Geometry: final body of the model. Coordinates: model frame, mm. A direction names the side the tool comes from. Give positions to 0.01 mm unless a question says otherwise; leave off trailing zeros. Loops run counter-clockwise (first coordinate to the right, second up) from the corner with the lowest first, then second, coordinate; pieces in that order, holes last. Notation, with made-up numbers: (54, 8) -> (111, 8) arc R25 cw to (111, 40) -> close; hole circle Ø4 at (-19.5, 64). An arc over 180 degrees is marked (long way). Answer in a Markdown table with one row per item. Add a question column.
1) Section query B-B (y = -2). Return the cut outline in (x, z), plus the area to 3 significant figures.
2) Section query D-D (y = 3.75). Return the cut outline in (x, z).
3) Section query A-A (z = 0). Return the cut outline in (x, y).
4) Draft query along X for faces 5 (the cylindrical face through (-0.217, 4.205, -7.276)), 6 (the flat face through (-1, 0, -8.9)), 7 (the cylindrical face through (-1.5, 0.04, 0.07)). Return one class per face: +X half, -X half, draft (parallel to the pull), parting line (faces both ways), or undercut.
5) Access query for faces 1 (the cylindrical face through (-0.217, -4.245, -7.276)), 2 (the flat face through (3, 0, -1)), 3 (the flat face through (1, 0, -10)), 4 (the flat face through (0, 0, 8)). Directions: +Z, -Z, +X, -X, +Y, -Y. A direction counts if a zero-diameter tool reaches every point of the face in a straight line with its end or side. Return the directions, or none.
6) Line query: line 1 (Y direction, x = -0.35, z = -1.5); line 2 (Z direction, x = -0.7, y = -0.75); line 3 (X direction, y = 0, z = -0.5). Output: solid intervals per line, ascending. Write a range as from..to.
7) Section query C-C (z = -6.3). Return the cut outline in (x, y).
8) First-contact query: P1, Ø3.5, axis at x = 0, z = 0, coming from the +Y side; P2, Ø3.5, axis at y = -1, z = 8.5, coming from the +X side; P3, Ø1, axis at x = -1, y = -2.5, coming from the +Z side. Flat tips, straight axial feed; report the tip coordinate or a pass-through.
```python
from build123d import *

# Parameters (mm, degrees)
F0_R     = 1
F0_R_2   = 1.5
F1_DEPTH = 2.8
F2_DEPTH = 5.65


with BuildPart() as f1:
    # F0 (on Front) → F1 (new body, symmetric)
    with BuildSketch(Plane.XZ):
        Polygon((0, 9.9), (-3, 6.9), (-3, -6.9), (1, -10.9), (1, -8.3), (3, -7.9), (3, 5.6), (0, 6.5), align=None)
        with Locations((0, -6.3)):
            Circle(F0_R, mode=Mode.SUBTRACT)
        Circle(F0_R_2, mode=Mode.SUBTRACT)
    extrude(amount=F1_DEPTH, both=True)

    # F0 (on Front) → F2 (join, symmetric)
    with BuildSketch(Plane.XZ):
        with Locations((0, -6.3)):
            Circle(F0_R)
    extrude(amount=F2_DEPTH, both=True)


solid = f1.part
```
Evaluation:
| question | item | result |
|---|---|---|
| 1 | outline | (-3, -6.9) -> (1, -10.9) -> (1, -8.3) -> (3, -7.9) -> (3, 5.6) -> (0, 6.5) -> (0, 9.9) -> (-3, 6.9) -> close; hole circle Ø3 at (0, 0) |
| 1 | area | 88.1 mm² |
| 2 | outline | circle Ø2 at (0, -6.3) |
| 3 | outline | (-3, -2.8) -> (-1.5, -2.8) -> (-1.5, 2.8) -> (-3, 2.8) -> close; (1.5, -2.8) -> (3, -2.8) -> (3, 2.8) -> (1.5, 2.8) -> close |
| 4 | face 5 | parting line |
| 4 | face 6 | -X half |
| 4 | face 7 | undercut |
| 5 | face 1 | -Y |
| 5 | face 2 | +Z, -Z, +X, +Y, -Y |
| 5 | face 3 | -Z, +X, +Y, -Y |
| 5 | face 4 | +Z, +X, +Y, -Y |
| 6 | line 1 | -2.8..2.8 |
| 6 | line 2 | -9.2..-1.33, 1.33..9.2 |
| 6 | line 3 | -3..-1.41, 1.41..3 |
| 7 | outline | (-3, -2.8) -> (-1, -2.8) -> (-1, -5.65) -> (1, -5.65) -> (1, -2.8) -> (3, -2.8) -> (3, 2.8) -> (1, 2.8) -> (1, 5.65) -> (-1, 5.65) -> (-1, 2.8) -> (-3, 2.8) -> close |
| 8 | P1 | y = 2.8 |
| 8 | P2 | x = 0 |
| 8 | P3 | z = 9.4 |
